Autodesk Inventor part; units mm, degrees
ref_plane "YZ Plane" through (0, 0, 0) normal (1, 0, 0) x (0, 1, 0)
ref_plane "XZ Plane" through (0, 0, 0) normal (0, 1, 0) x (-1, 0, 0)
ref_plane "XY Plane" through (0, 0, 0) normal (0, 0, 1) x (1, 0, 0)
sketch "Sketch1" plane through (0, 0, 0) normal (0, 1, 0) x (-1, 0, 0)
  line L0 (18.923, 65.405) -> (-18.923, 65.405)
  line L1 (-18.923, 65.405) -> (-18.923, -65.405)
  line L2 (-18.923, -65.405) -> (18.923, -65.405)
  line L3 (18.923, -65.405) -> (18.923, 65.405)
  line L4 (18.923, 65.405) -> (-18.923, -65.405) construction
  line L5 (-18.923, 65.405) -> (18.923, -65.405) construction
  line L6 (20.828, 67.31) -> (-20.828, 67.31)
  line L7 (-20.828, 67.31) -> (-20.828, -67.31)
  line L8 (-20.828, -67.31) -> (20.828, -67.31)
  line L9 (20.828, -67.31) -> (20.828, 67.31)
  point P0 (0, 0)
  dimension "d0" = 37.846
  dimension "d1" = 130.81
  dimension "d2" = 1.905
extrude "Extrusion1" add sketch "Sketch1" along normal blind 20.32
extrude "Extrusion2" add sketch "Sketch1" along normal blind 1.905 contours L3 L2 L1 L0
sketch "Sketch2" plane through (20.828, 0, 67.31) normal (1, 0, 0) x (0, 0, -1)
  line L0 (12.7, 20.32) -> (121.92, 20.32)
  line L1 (121.92, 20.32) -> (121.92, 7.62)
  line L2 (121.92, 7.62) -> (12.7, 7.62)
  line L3 (12.7, 7.62) -> (12.7, 20.32)
  line L4 (0, 0) -> (0, 20.32)
  line L5 (134.62, 0) -> (134.62, 20.32)
  line L6 (0, 20.32) -> (134.62, 20.32)
  line L7 (0, 0) -> (134.62, 0)
  point P0 (67.31, 0)
  dimension "d7" = 12.7
  dimension "d8" = 12.7
  dimension "d9" = 7.62
extrude "Extrusion3" cut sketch "Sketch2" against normal blind 1.905 contours L0 L1 L2 L3
sketch "Sketch3" plane through (-20.828, 0, -67.31) normal (-1, 0, 0) x (0, 0, 1)
  line L0 (12.7, 20.32) -> (121.92, 20.32)
  line L1 (121.92, 20.32) -> (121.92, 5.08)
  line L2 (121.92, 5.08) -> (12.7, 5.08)
  line L3 (12.7, 5.08) -> (12.7, 20.32)
  line L4 (0, 20.32) -> (134.62, 20.32)
  line L5 (0, 0) -> (0, 20.32)
  line L6 (134.62, 0) -> (134.62, 20.32)
  line L7 (0, 0) -> (134.62, 0)
  point P0 (67.31, 0)
  dimension "d12" = 12.7
  dimension "d13" = 12.7
  dimension "d14" = 5.08
extrude "Extrusion4" cut sketch "Sketch3" against normal blind 1.905 contours L0 L1 L2 L3
sketch "Sketch4" plane through (0, 20.32, 0) normal (0, 1, 0) x (1, 0, 0)
  line L0 (20.828, 67.31) -> (-20.828, 67.31)
  line L1 (-18.923, 65.405) -> (18.923, 65.405)
  line L2 (13.843, 67.31) -> (11.557, 67.31)
  line L3 (11.557, 67.31) -> (11.557, 65.405)
  line L4 (11.557, 65.405) -> (13.843, 65.405)
  line L5 (13.843, 65.405) -> (13.843, 67.31)
  line L6 (18.923, 65.405) -> (18.923, 54.61)
  line L7 (-18.923, 54.61) -> (-18.923, 65.405)
  point P0 (0, 0)
  dimension "d17" = 5.08
  dimension "d18" = 30.48
extrude "Extrusion5" cut sketch "Sketch4" against normal up to surface (18.415 mm away)
sketch "Sketch5" plane through (20.828, 0, -67.31) normal (0, 0, -1) x (-1, 0, 0)
  line L0 (0, 0) -> (41.656, 0)
  line L1 (0, 0) -> (41.656, 0)
  line L2 (41.656, 0) -> (41.656, 1.905)
  line L3 (41.656, 1.905) -> (0, 1.905)
  line L4 (0, 1.905) -> (0, 0)
  line L5 (9.271, 1.905) -> (6.985, 1.905)
  line L6 (41.656, 0) -> (41.656, 20.32)
  point P0 (20.828, 0)
extrude "Extrusion6" add sketch "Sketch5" along normal blind 24.13
sketch "Sketch6" plane through (0, 1.905, 0) normal (0, 1, 0) x (1, 0, 0)
  line L0 (-19.177, 76.835) -> (4.445, 76.835)
  line L1 (4.445, 76.835) -> (4.445, 89.789)
  line L2 (4.445, 89.789) -> (-19.177, 89.789)
  line L3 (-19.177, 89.789) -> (-19.177, 76.835)
  line L4 (18.923, 65.405) -> (18.923, 54.61)
  line L5 (11.557, 67.31) -> (-20.828, 67.31)
  line L6 (-20.828, 75.184) -> (6.096, 75.184)
  line L7 (6.096, 75.184) -> (6.096, 91.44)
  line L8 (6.096, 91.44) -> (-20.828, 91.44)
  line L9 (-20.828, 91.44) -> (-20.828, 75.184)
  line L10 (-20.828, 91.44) -> (20.828, 91.44)
  line L11 (-20.828, 67.31) -> (-20.828, 91.44)
  line L12 (-18.923, 65.405) -> (11.557, 65.405)
  point P0 (0, 0)
  dimension "d24" = 12.954
  dimension "d26" = 23.622
  dimension "d32" = 11.43
extrude "Extrusion7" add sketch "Sketch6" along normal blind 33.02
sketch "Sketch8" plane through (4.445, 1.905, -89.789) normal (-1, 0, 0) x (0, 0, 1)
  circle A0 centre (6.477, 20.32) radius 6.477
  line L0 (0, 0) -> (0, 33.02)
  line L1 (12.954, 0) -> (12.954, 33.02)
  line L2 (0, 0) -> (12.954, 0)
  line L3 (12.954, 20.32) -> (12.954, 33.02)
  line L4 (0, 33.02) -> (0, 20.32)
  line L5 (12.954, 33.02) -> (0, 33.02)
  line L6 (12.954, 20.32) -> (12.954, 33.02)
  line L7 (0, 33.02) -> (0, 20.32)
  point P0 (89.789, -1.905)
  dimension "d29" = 20.32
extrude "Extrusion8" cut sketch "Sketch8" against normal blind 33.02 contours A0 | A0 L0 L5 L1
sketch "Sketch10" plane through (4.445, 1.905, -89.789) normal (-1, 0, 0) x (0, 0, 1)
  line L0 (-1.651, 0) -> (14.605, 0)
  line L1 (-1.651, 0) -> (-1.651, 33.02)
  line L2 (14.605, 0) -> (-1.651, 0)
  line L3 (-1.651, 0) -> (-1.651, 13.208)
  line L4 (-1.651, 13.208) -> (14.605, 13.208)
  line L5 (14.605, 13.208) -> (14.605, 0)
  arc A0 (0, 20.32) -> (12.954, 20.32) centre (6.477, 20.32) ccw
  point P0 (89.789, -1.905)
  point P1 (6.477, 13.843)
  point P2 (6.477, 13.208)
  dimension "d37" = 0.635
extrude "Extrusion10" add sketch "Sketch10" along normal blind 3.048
sketch "Sketch9" plane through (6.096, 1.905, -75.184) normal (1, 0, 0) x (0, 0, -1)
  arc A0 (1.651, 20.32) -> (14.605, 20.32) centre (8.128, 20.32) ccw
  circle A1 centre (8.372, 11.303) radius 1.524
  point P0 (-75.184, -1.905)
  point P1 (8.128, 13.843)
  dimension "d33" = 2.54
  dimension "d34" = 3.048
extrude "Extrusion9" cut sketch "Sketch9" against normal up to surface (25.273 mm away)
sketch "Sketch11" plane through (20.828, 0, 67.31) normal (1, 0, 0) x (0, 0, -1)
  line L0 (134.62, 1.905) -> (158.75, 1.905)
  line L1 (0, 0) -> (158.75, 0)
  line L2 (158.75, 0) -> (158.75, 1.905)
  line L3 (158.75, 1.905) -> (0, 1.905)
  line L4 (0, 1.905) -> (0, 0)
  point P0 (67.31, 0)
extrude "Extrusion11" add sketch "Sketch11" along normal blind 76.2
sketch "Sketch12" plane through (0, 1.905, 0) normal (0, 1, 0) x (1, 0, 0)
  circle A0 centre (90.678, -43.815) radius 3.81
  line L0 (20.828, 54.61) -> (20.828, -54.61)
  line L1 (18.923, -65.405) -> (-18.923, -65.405)
  line L2 (20.828, -51.435) -> (97.028, -51.435)
  line L3 (97.028, 91.44) -> (97.028, -67.31)
  line L4 (97.028, -67.31) -> (20.828, -67.31)
  line L5 (20.828, -67.31) -> (20.828, -51.435)
  line L6 (97.028, -36.195) -> (20.828, -36.195)
  line L7 (-20.828, 91.44) -> (97.028, 91.44)
  line L8 (20.828, 91.44) -> (97.028, 91.44)
  line L9 (97.028, 91.44) -> (97.028, -36.195)
  line L10 (20.828, -36.195) -> (97.028, -36.195)
  line L11 (97.028, -36.195) -> (97.028, 91.44)
  line L12 (97.028, 91.44) -> (20.828, 91.44)
  line L13 (20.828, 91.44) -> (20.828, -36.195)
  line L14 (6.096, 91.44) -> (97.028, 91.44)
  line L15 (97.028, 91.44) -> (97.028, 67.31)
  line L16 (6.096, 67.31) -> (6.096, 91.44)
  line L17 (6.096, 89.789) -> (6.096, 91.44)
  line L18 (20.828, 67.31) -> (13.843, 67.31)
  circle A1 centre (65.278, -34.29) radius 3.81
  circle A2 centre (90.678, -24.765) radius 3.81
  circle A3 centre (90.678, -5.715) radius 3.81
  circle A4 centre (90.678, 13.335) radius 3.81
  circle A5 centre (90.678, 32.385) radius 3.81
  circle A6 centre (65.278, -15.24) radius 3.81
  circle A7 centre (65.278, 3.81) radius 3.81
  circle A8 centre (65.278, 22.86) radius 3.81
  circle A9 centre (65.278, 41.91) radius 3.81
  line L19 (20.828, 91.44) -> (97.028, 91.44)
  line L20 (97.028, 91.44) -> (97.028, 49.53)
  line L21 (97.028, 49.53) -> (20.828, 49.53)
  line L22 (20.828, 49.53) -> (20.828, 91.44)
  line L23 (6.096, 67.31) -> (20.828, 67.31)
  line L24 (20.828, 67.31) -> (20.828, 91.44)
  line L25 (20.828, 91.44) -> (6.096, 91.44)
  line L26 (6.096, 91.44) -> (6.096, 67.31)
  point P0 (0, 0)
  point P1 (97.028, -36.195)
  point P2 (20.828, -54.61)
  point P3 (6.096, 90.5705)
  point P4 (5.715, 89.789)
  point P5 (20.828, 49.53)
  dimension "d42" = 7.62
  dimension "d44" = 21.59
  dimension "d45" = 7.62
  dimension "d46" = 7.62
  dimension "d59" = 7.62
  dimension "d76" = 69.85
  dimension "d79" = 19.05
  dimension "d84" = 9.525
  dimension "d87" = 19.05
  dimension "d92" = 25.4
  dimension "d93" = 7.62
extrude "Extrusion12" cut sketch "Sketch12" against normal blind 57.15 contours A0 | L13 L7 L3 L21 L0 | L18 L23 L16 L7 L13 | L2 L3 L4 L5 L0 | A1 L6 | L6 A1 | A2 | A3 | A4 | A5 | A6 | A7 | A8 | A9
sketch "Sketch13" plane through (0, 1.905, 0) normal (0, 1, 0) x (1, 0, 0)
  line L0 (11.557, 67.31) -> (-20.828, 67.31)
  line L1 (-20.828, 75.184) -> (6.096, 75.184)
  line L2 (-13.208, 67.31) -> (-1.524, 67.31)
  line L3 (-1.524, 67.31) -> (-1.524, 75.184)
  line L4 (-1.524, 75.184) -> (-13.208, 75.184)
  line L5 (-13.208, 75.184) -> (-13.208, 67.31)
  line L6 (-20.828, 67.31) -> (-20.828, 75.184)
  line L7 (6.096, 91.44) -> (6.096, 75.184)
  point P0 (0, 0)
  point P1 (-20.828, 71.247)
  point P2 (-13.208, 71.247)
  point P3 (6.096, 67.31)
  point P4 (-1.524, 67.31)
  point P5 (-13.208, 75.184)
  point P6 (-1.524, 67.31)
  dimension "d49" = 7.62
  dimension "d50" = 7.62
extrude "Extrusion13" add sketch "Sketch13" along normal blind 12.7
sketch "Sketch15" plane through (-19.177, 1.905, -76.835) normal (1, 0, 0) x (0, 0, -1)
  line L0 (0, 0) -> (12.954, 0)
  line L1 (12.954, 0) -> (12.954, 6.35)
  line L2 (12.954, 6.35) -> (0, 6.35)
  line L3 (0, 6.35) -> (0, 0)
  line L4 (-144.145, -1.905) -> (14.605, -1.905)
  line L5 (14.605, -1.905) -> (14.605, 33.02)
  point P0 (-76.835, -1.905)
  dimension "d94" = 12.954
  dimension "d95" = 6.35
  dimension "d96" = 1.905
  dimension "d97" = 1.651
extrude "Extrusion14" cut sketch "Sketch15" against normal blind 57.15
properties part number "HarmonicaFrame2"
Build history of the part. All positions in model axes, mm. A direction names the side the tool comes from. Give positions to 0.01 mm unless a question says otherwise; leave off trailing zeros. Order: outer loops, then holes, each group sorted by start corner. A loop starts at its lowest first (then second) coordinate and runs counter-clockwise, first axis right, second up. Notation, with made-up numbers: M 43.5,-40 L 79.5,-40 A21 cw 79.5,-7 Z; hole C 15,9 d8. An arc over 180 degrees is marked long. Put each result on its own line as item: value.
Item 1: Flat gauge pins, fed straight in: pin 1 Ø2.5 at (x, z) = (2.5, -82.5) entering from +Y; pin 2 Ø0.6 at (x, z) = (20.5, 5) entering from +Y; pin 3 Ø8 at (x, y) = (58.5, 7.5) entering from -Z; pin 4 Ø0.6 at (x, y) = (67, 1.5) entering from +Z (3 decimals). Where does each tip first touch, or does it go through?
From the geometry:
pin 1: stops at y = 15.11
pin 2: stops at y = 7.62
pin 3: passes through
pin 4: stops at z = 51.435
Item 2: Slice it at A-A, the plane z = 15.24. Write the cut outline in (x, y) (3 decimals), plus the area to 3 significant figures.
From the geometry:
outline: M -20.828,0 L 61.468,0 L 61.468,1.905 L 20.828,1.905 L 20.828,7.62 L 18.923,7.62 L 18.923,1.905 L -18.923,1.905 L -18.923,5.08 L -20.828,5.08 Z; M 69.088,0 L 97.028,0 L 97.028,1.905 L 69.088,1.905 Z
area: 227 mm2
Item 3: Slice it at B-B, the plane y = 32. Write the cut outline in (x, z) (3 decimals).
From the geometry:
outline: M -20.828,-91.44 L 6.096,-91.44 L 6.096,-89.789 L -19.177,-89.789 L -19.177,-76.835 L 6.096,-76.835 L 6.096,-75.184 L -20.828,-75.184 Z
Item 4: 3-axis set-ups, long thin cutter, end or side, ignore diameter. For faces 1 (the flat face through (-8, 17, -91.44)), 2 (the flat face through (-5, 22, -75.184)), 3 (the flat face through (16, 11, -65.405)), 4 (the flat face through (-11, 14.605, -71)): which of +Z, -Z, +X, -X, +Y, -Y reach the whole face in a straight line?
From the geometry:
face 1: -Z, +X, -X, +Y, -Y
face 2: +X, +Y
face 3: +Y
face 4: +X, -X, +Y
Item 5: Slice it at D-D, the plane z = -71. Write the cut outline in (x, y) (3 decimals), plus the area to 3 significant figures.
From the geometry:
outline: M -20.828,0 L 6.096,0 L 6.096,1.905 L -1.524,1.905 L -1.524,14.605 L -20.828,14.605 Z
area: 296 mm2
Item 6: Probe line 1 (Z direction, x = -14.5, y = 8.5) (3 decimals); line 2 (Z direction, x = -13, y = 20.5) (3 decimals); line 3 (X direction, y = 8, z = -57). List the from-to ranges inside material, lowest first. Write a range as [from, to].
From the geometry:
line 1: z = [-91.44, -89.789], [-76.835, -65.405], [65.405, 67.31]
line 2: z = [-91.44, -89.789], [-76.835, -75.184]
line 3: x = [-20.83, -18.92], [18.92, 20.83]
Item 7: Two-plate mould, pull along X, no slides. Class faces 5 (the cylindrical face through (94.31, 0.97, 23.62)), 6 (the flat face through (58, 1.905, 2)), 7 (the flat face through (20.828, 6, 1)): +X half, -X half, draft (parallel to the pull), parting line (faces both ways), or undercut.
From the geometry:
face 5: undercut
face 6: draft
face 7: +X half
Item 8: Slice it at C-C, the plane x = 39. Write the cut outline in (y, z) (3 decimals).
From the geometry:
outline: M 0,-49.53 L 1.905,-49.53 L 1.905,51.435 L 0,51.435 Z
